Source: CAD feature listing. Evaluate the final solid. Frame: model axes, mm. A direction names the side the tool comes from. Coordinates: 2 decimals unless noted, no trailing zeros. Loops run counter-clockwise (first coordinate to the right, second up) from the corner with the lowest first, then second, coordinate; pieces in that order, holes last. Notation, with made-up numbers: (-17.75, 59.25) - (37.25, 59.25) arc R23 cw to (37.25, 86.25) - close; hole circle Ø8 at (8.5, 80.25). An arc over 180 degrees is marked (long way). Use one line per item in the form item = value. Start each with the question number.
Autodesk Inventor part; units mm, degrees
ref_plane "YZ Plane" through (0, 0, 0) normal (1, 0, 0) x (0, 1, 0)
ref_plane "XZ Plane" through (0, 0, 0) normal (0, 1, 0) x (-1, 0, 0)
ref_plane "XY Plane" through (0, 0, 0) normal (0, 0, 1) x (1, 0, 0)
sketch "Sketch1" plane through (0, 0, 0) normal (0, 0, 1) x (1, 0, 0)
  line L0 (0, 0) -> (43, 0)
  line L1 (43, 0) -> (43, 9)
  line L2 (43, 9) -> (0, 9)
  line L3 (0, 9) -> (0, 0)
  dimension "d0" = 43
  dimension "d1" = 9
extrude "Extrusion1" add sketch "Sketch1" along normal blind 5
sketch "Sketch2" plane through (0, 0, 5) normal (0, 0, 1) x (1, 0, 0)
  line L0 (43, 0) -> (43, 9)
  line L1 (43, 9) -> (0, 9)
  point P0 (0, 0)
  point P1 (35.7, 4.5)
  point P2 (6.2, 4.5)
  dimension "d11" = 7.3
  dimension "d12" = 29.5
  dimension "d13" = 4.5
  dimension "d14" = 4.5
hole "Hole1" at (35.7, 4.5, 5) at (6.2, 4.5, 5) direction (0, 0, -1) diameter 3.3 end through all
sketch "Sketch3" plane through (0, 0, 5) normal (0, 0, 1) x (1, 0, 0)
  line L0 (0, 0) -> (43, 0)
  line L1 (43, 9) -> (0, 9)
  line L2 (9.7, 0) -> (12.2, 0)
  line L3 (12.2, 0) -> (12.2, 9)
  line L4 (12.2, 9) -> (9.7, 9)
  line L5 (9.7, 9) -> (9.7, 0)
  line L6 (29.7, 9) -> (32.2, 9)
  line L7 (32.2, 9) -> (32.2, 0)
  line L8 (32.2, 0) -> (29.7, 0)
  line L9 (29.7, 0) -> (29.7, 9)
  circle A0 centre (35.7, 4.5) radius 1.65
  point P0 (29.7, 4.5)
  point P1 (12.2, 4.5)
  point P2 (32.2, 4.5)
  point P3 (29.7, 9)
  point P4 (29.7, 0)
  point P5 (32.2, 0)
  point P6 (32.2, 9)
  point P7 (12.2, 0)
  dimension "d15" = 2.5
  dimension "d16" = 2.5
  dimension "d17" = 17.5
  dimension "d18" = 3.5
extrude "Extrusion2" add sketch "Sketch3" along normal blind 30 contours L5 L1 L3 L0 | L9 L1 L7 L0
sketch "Sketch6" plane through (0, 9, 0) normal (0, 1, 0) x (1, 0, 0)
  line L0 (12.2, -5) -> (12.2, -35)
  line L1 (12.2, -30) -> (9.7, -30)
  line L2 (12.2, -33) -> (9.7, -33)
  line L3 (9.7, -33) -> (9.7, -30)
  line L4 (9.7, -30) -> (12.2, -30)
  line L5 (12.2, -30) -> (12.2, -33)
  line L6 (29.7, -5) -> (29.7, -35)
  line L7 (29.7, -30) -> (32.2, -30)
  line L8 (32.2, -30) -> (32.2, -33)
  line L9 (32.2, -33) -> (29.7, -33)
  line L10 (29.7, -33) -> (29.7, -30)
  point P0 (0, 0)
  dimension "d30" = 2.5
  dimension "d31" = 3
  dimension "d32" = 3
extrude "Extrusion5" add sketch "Sketch6" along normal blind 28
sketch "Sketch7" plane through (29.7, 0, 5) normal (-1, 0, 0) x (0, 0, 1)
  line L0 (25, 37) -> (28, 37)
  line L1 (28, 37) -> (25, 37)
  line L2 (25, 37) -> (25, 34)
  line L3 (25, 34) -> (28, 34)
  line L4 (28, 34) -> (28, 37)
  point P0 (-5, 0)
  dimension "d35" = 3
  dimension "d36" = 3
extrude "Extrusion6" add sketch "Sketch7" along normal blind 18
properties part number "Batteryholder1"
(1) Material intervals for line 1 (X direction, y = 4.5, z = 3.3); line 2 (Y direction, x = 35.7, z = 3.1); line 3 (Z direction, x = 11.5, y = 26), sorted ascending.
(2) Access query for faces 1 (the face through (20.2, 34.3, 33)), 2 (the face through (21, 5, 5)), 3 (the face through (21, 34.5, 30)). Directions: +Z, -Z, +X, -X, +Y, -Y. A direction counts if a zero-diameter tool reaches every point of the face in a straight line with its end or side. Return the directions, or none.
(3) Cut plane C-C, the plane y = 4.5. Output: boundary loops of the cut face in (x, z), plus the area to 3 significant figures.
(4) Cut plane D-D, the plane x = 11. Output: boundary loops of the cut face in (y, z).
(5) Mould query, pull axis X, two halves, no side actions, for faces 4 (the face through (9.7, 8, 21)), 5 (the face through (12.2, 7, 22)), 6 (the face through (21, 37, 31)). Classes: +X half, -X half, draft (parallel to the pull), parting line (faces both ways), or undercut.
(6) Contact query for flat-ended pins moving along their axis: pin 1 (12 mm diameter, centred on y = 27, z = 31, fed in from -X); pin 2 (1 mm diameter, centred on x = 11.5, z = 34, fed in from +Y); pin 3 (18 mm diameter, centred on x = 22, y = 26.5, fed in from -Z). Output: stop coordinate, or through.
(7) Cut plane A-A, the plane z = 12.5. Output: boundary loops of the cut face in (x, y).
(8) Cut plane B-B, the plane y = 22. Output: boundary loops of the cut face in (x, z).
Recorded:
q1.line_1 = 0 to 4.55, 7.85 to 34.05, 37.35 to 43
q1.line_2 = 0 to 2.85, 6.15 to 9
q1.line_3 = 30 to 33
q2.face_1 = +Z, +X, -X, +Y
q2.face_2 = +Z, +Y, -Y
q2.face_3 = -Z, +X, -X, +Y
q3.outline = (0, 0) - (4.55, 0) - (4.55, 5) - (0, 5) - close; (7.85, 0) - (34.05, 0) - (34.05, 5) - (32.2, 5) - (32.2, 35) - (29.7, 35) - (29.7, 5) - (12.2, 5) - (12.2, 35) - (9.7, 35) - (9.7, 5) - (7.85, 5) - close; (37.35, 0) - (43, 0) - (43, 5) - (37.35, 5) - close
q3.area = 332 mm²
q4.outline = (0, 0) - (9, 0) - (9, 30) - (37, 30) - (37, 33) - (9, 33) - (9, 35) - (0, 35) - close
q5.face_4 = -X half
q5.face_5 = undercut
q5.face_6 = draft
q6.pin_1 = 9.7
q6.pin_2 = 9
q6.pin_3 = 30
q7.outline = (9.7, 0) - (12.2, 0) - (12.2, 9) - (9.7, 9) - close; (29.7, 0) - (32.2, 0) - (32.2, 9) - (29.7, 9) - close
q8.outline = (9.7, 30) - (12.2, 30) - (12.2, 33) - (9.7, 33) - close; (29.7, 30) - (32.2, 30) - (32.2, 33) - (29.7, 33) - close
